Geometry: final body of the model. Coordinates: model frame, mm. A direction names the side the tool comes from. Round coordinates to 2 decimals unless told otherwise and drop trailing zeros. Write each loop counter-clockwise with the first axis right and the second up, starting at its lowest first coordinate (ties: lowest second). Pieces come first, ordered by that corner, then holes. Notation, with made-up numbers: (-27, 79.5) -> (18, 79.5) arc R9 cw to (18, 96.5) -> close; hole circle Ø10 at (20.5, -18.75). An arc over 180 degrees is marked (long way). Use one line per item in the form item = value. Start each with the question number.
1. Cut plane D-D, the plane y = -16.5. Return the cut outline in (x, z).
2. Reachability of faces 1 (the face through (0, -17, 0)), 2 (the face through (0, 0, -3)), 3 (the face through (-1.344, -3.944, 2.191)) from +Z, -Z, +X, -X, +Y, -Y: full face, straight path, thin tool, end or side. Return the list, or none.
3. Pin query (flat end, axial travel): pin 1 Ø8 at (y, z) = (-7, 1.5) entering from +X; pin 2 Ø5 at (x, y) = (-7.5, -11) entering from +Z; pin 3 Ø6 at (y, z) = (-16, 7) entering from +X; pin 4 Ø5 at (x, z) = (-3, 0.5) entering from -Y. Return the tip coordinate at first contact, or that it passes through.
4. Draft query along Z for faces 4 (the face through (0, -8, 0)), 5 (the face through (11.923, -12.325, 3.755)), 6 (the face through (-0.2, -25, -8.2)), 7 (the face through (-1.73, -21.06, -7.81)). Return one class per face: pulls with the +Z half, pulls with the -Z half, needs draft (parallel to the pull), parting line crosses it, or undercut.
5. Line query: L1, parallel to Z at x = 0, y = -22.25; L2, parallel to Z at x = 0, y = -4.5. Output: solid intervals per line, ascending.
6. Cut plane B-B, the plane y = -23.25. Return the cut outline in (x, z).
7. Cut plane C-C, the plane z = -1.5. Return the cut outline in (x, y), plus the area to 3 significant figures.
8. Cut plane A-A, the plane x = 0. Return the cut outline in (y, z), plus the area to 3 significant figures.
```python
from build123d import *

# Parameters (mm, degrees)
F0_R     = 12.5
F1_DEPTH = 25
F2_R     = 2.5
F3_DEPTH = 8
F4_R     = 8
F5_DEPTH = 8


with BuildPart() as f1:
    # F0 (on Front) → F1 (new body)
    with BuildSketch(Plane.XZ):
        Circle(F0_R)
    extrude(amount=F1_DEPTH)

    # F2 (on face) → F3 (cut)
    with BuildSketch(Plane(origin=(0, 0, 0), x_dir=(-1, 0, 0), z_dir=(0, 1, 0))):
        with Locations((0, 0.083146)):
            Circle(F2_R)
    extrude(amount=-F3_DEPTH, mode=Mode.SUBTRACT)

    # F4 (on face) → F5 (cut)
    with BuildSketch(Plane.XZ.offset(25)):
        Circle(F4_R)
    extrude(amount=-F5_DEPTH, mode=Mode.SUBTRACT)


solid = f1.part
```
Outcome:
q1.outline = circle Ø25 at (0, 0)
q2.face_1 = -Y
q2.face_2 = +Z, -Z, +X, -X, +Y
q2.face_3 = +Y
q3.pin_1 = 12.5
q3.pin_2 = 11.46
q3.pin_3 = 11.84
q3.pin_4 = -17
q4.face_4 = undercut
q4.face_5 = parting line crosses it
q4.face_6 = needs draft
q4.face_7 = undercut
q5.L1 = -12.5 to -8, 8 to 12.5
q5.L2 = -12.5 to -2.42, 2.58 to 12.5
q6.outline = circle Ø25 at (0, 0); hole circle Ø16 at (0, 0)
q7.outline = (-12.41, -25) -> (-7.86, -25) -> (-7.86, -17) -> (7.86, -17) -> (7.86, -25) -> (12.41, -25) -> (12.41, 0) -> (1.93, 0) -> (1.93, -8) -> (-1.93, -8) -> (-1.93, 0) -> (-12.41, 0) -> close
q7.area = 464 mm^2
q8.outline = (-25, -12.5) -> (0, -12.5) -> (0, -2.42) -> (-8, -2.42) -> (-8, 2.58) -> (0, 2.58) -> (0, 12.5) -> (-25, 12.5) -> (-25, 8) -> (-17, 8) -> (-17, -8) -> (-25, -8) -> close
q8.area = 457 mm^2
